Can you work these out from the drawing? Everything is in mm from the part's minimum corner. Coordinates: 2 decimals unless noted, no trailing zeros. Order: outer loops, then holes, each group sorted by start corner. A loop starts at its lowest first (then second) coordinate and runs counter-clockwise, first axis right, second up. Notation, with made-up numbers: M -27.5,83.5 L 18.5,83.5 A7 ccw 18.5,89.5 Z; hole C 31,45 d2. An arc over 180 degrees is marked long. Answer as CSV lines item,"result". Start each with the question number.
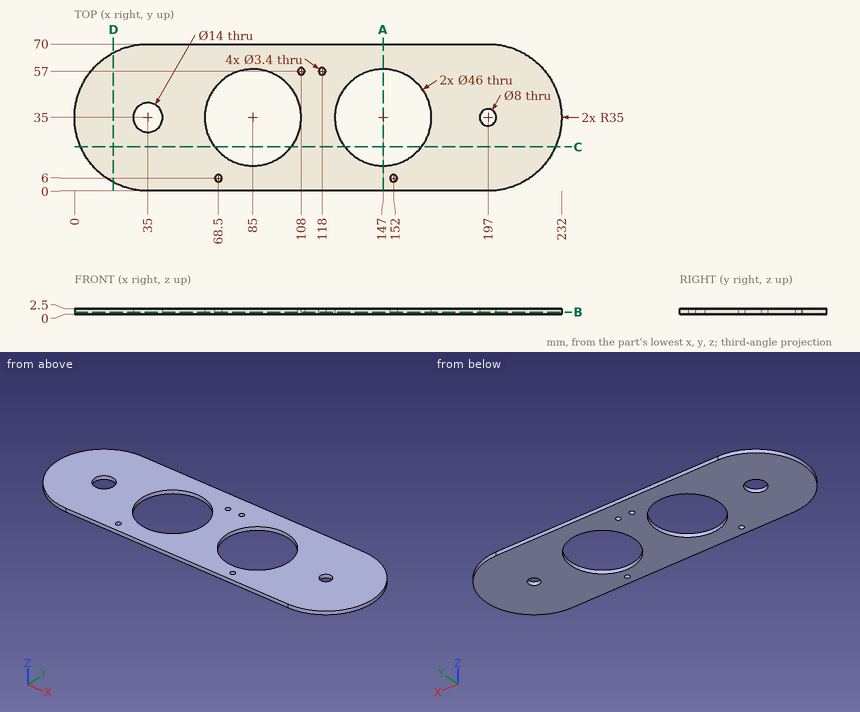
1) Suppose I cut it at C-C on y = 21. Please give me the cut outline in (x, z), plus the area to 3 significant figures.
2) Suppose I cut it at D-D on x = 18.5. Please give me the cut outline in (y, z).
3) I need wall thicknesses on line 1 (Y direction, x = 35, z = 1.4); line 2 (X direction, y = 38.5, z = 0.35); line 3 (X direction, y = 44, z = 0.5). Which ranges of each line are inside material? Lowest first, please. Write a range as [from, to].
4) Suppose I cut it at A-A on x = 147. Please give me the cut outline in (y, z), plus the area to 3 significant figures.
5) Suppose I cut it at B-B on z = 1. Give the number of separate pieces and of enclosed holes in the cut face, plus the area to 3 significant figures.
Output:
1,outline,"M 2.92,0 L 66.75,0 L 66.75,2.5 L 2.92,2.5 Z; M 103.25,0 L 128.75,0 L 128.75,2.5 L 103.25,2.5 Z; M 165.25,0 L 229.08,0 L 229.08,2.5 L 165.25,2.5 Z"
1,area,"383 mm²"
2,outline,"M 4.13,0 L 65.87,0 L 65.87,2.5 L 4.13,2.5 Z"
3,line 1,"[0, 28], [42, 70]"
3,line 2,"[0.18, 28.94], [41.06, 62.27], [107.73, 124.27], [169.73, 195.06], [198.94, 231.82]"
3,line 3,"[1.18, 63.83], [106.17, 125.83], [168.17, 230.82]"
4,outline,"M 0,0 L 12,0 L 12,2.5 L 0,2.5 Z; M 58,0 L 70,0 L 70,2.5 L 58,2.5 Z"
4,area,"60.0 mm²"
5,separate pieces,"1"
5,enclosed holes,"8"
5,area,"11,600 mm²"
